```python
from build123d import *

# Parameters (mm, degrees)
F0_W     = 2
F0_H     = 5
F0_W_2   = 47
F0_H_2   = 30
F1_DEPTH = 24
F2_W     = 40
F2_H     = 16
F3_DEPTH = 4
F4_W     = 40
F4_H     = 16
F5_DEPTH = 4
F6_R     = 1.65
F7_DEPTH = 25
F8_R     = 3
F9_DEPTH = 2


with BuildPart() as f1:
    # F0 (on Top) → F1 (new body)
    with BuildSketch(Plane.XY):
        with BuildLine():
            Line((28.5, 14.5), (28.5, 20))
            Line((28.5, 20), (-28.5, 20))
            Line((-28.5, 20), (-28.5, 14.5))
            ThreePointArc((-28.5, 14.5), (-28.646447, 14.146447), (-29, 14))
            Line((-29, 14), (-32.5, 14))
            Line((-32.5, 14), (-32.5, 5))
            Line((-32.5, 5), (-29, 5))
            ThreePointArc((-29, 5), (-28.646447, 4.853553), (-28.5, 4.5))
            Line((-28.5, 4.5), (-28.5, -4.5))
            ThreePointArc((-28.5, -4.5), (-28.646447, -4.853553), (-29, -5))
            Line((-29, -5), (-32.5, -5))
            Line((-32.5, -5), (-32.5, -14))
            Line((-32.5, -14), (-29, -14))
            ThreePointArc((-29, -14), (-28.646447, -14.146447), (-28.5, -14.5))
            Line((-28.5, -14.5), (-28.5, -20))
            Line((-28.5, -20), (28.5, -20))
            Line((28.5, -20), (28.5, -14.5))
            ThreePointArc((28.5, -14.5), (28.646447, -14.146447), (29, -14))
            Line((29, -14), (32.5, -14))
            Line((32.5, -14), (32.5, -5))
            Line((32.5, -5), (29, -5))
            ThreePointArc((29, -5), (28.646447, -4.853553), (28.5, -4.5))
            Line((28.5, -4.5), (28.5, 4.5))
            ThreePointArc((28.5, 4.5), (28.646447, 4.853553), (29, 5))
            Line((29, 5), (32.5, 5))
            Line((32.5, 5), (32.5, 14))
            Line((32.5, 14), (29, 14))
            ThreePointArc((29, 14), (28.646447, 14.146447), (28.5, 14.5))
        make_face()
        with Locations((-29.5, -9.5)):
            Rectangle(F0_W, F0_H, mode=Mode.SUBTRACT)
        with Locations((29.5, -9.5)):
            Rectangle(F0_W, F0_H, mode=Mode.SUBTRACT)
        with Locations((-29.5, 9.5)):
            Rectangle(F0_W, F0_H, mode=Mode.SUBTRACT)
        Rectangle(F0_W_2, F0_H_2, mode=Mode.SUBTRACT)
        with Locations((29.5, 9.5)):
            Rectangle(F0_W, F0_H, mode=Mode.SUBTRACT)
    extrude(amount=F1_DEPTH)

    # F2 (on face) → F3 (cut)
    with BuildSketch(Plane(origin=(-32.5, 0, 0), x_dir=(0, -1, 0), z_dir=(-1, 0, 0))):
        with Locations((0, 12)):
            Rectangle(F2_W, F2_H)
    extrude(amount=-F3_DEPTH, mode=Mode.SUBTRACT)

    # F4 (on face) → F5 (cut)
    with BuildSketch(Plane.YZ.offset(32.5)):
        with Locations((0, 12)):
            Rectangle(F4_W, F4_H)
    extrude(amount=-F5_DEPTH, mode=Mode.SUBTRACT)

    # F6 (on face) → F7 (cut)
    with BuildSketch(Plane.XZ.offset(-15)):
        with Locations((-5, 19)):
            Circle(F6_R)
        with Locations((-5, 5)):
            Circle(F6_R)
        with Locations((5, 19)):
            Circle(F6_R)
        with Locations((5, 5)):
            Circle(F6_R)
    extrude(amount=-F7_DEPTH, mode=Mode.SUBTRACT)

    # F8 (on face) → F9 (cut)
    with BuildSketch(Plane.XZ.offset(-15)):
        with Locations((-5, 19)):
            Circle(F8_R)
        with Locations((-5, 5)):
            Circle(F8_R)
        with Locations((5, 19)):
            Circle(F8_R)
        with Locations((5, 5)):
            Circle(F8_R)
    extrude(amount=-F9_DEPTH, mode=Mode.SUBTRACT)


solid = f1.part
```
Can you work these out from the model? Positions are in its coordinate system, mm. A direction names the side the tool comes from. Round coordinates to 2 decimals unless told otherwise and drop trailing zeros. Loops run counter-clockwise (first coordinate to the right, second up) from the corner with the lowest first, then second, coordinate; pieces in that order, holes last. Notation, with made-up numbers: M 49.5,35.5 L 73.5,35.5 A31 ccw 73.5,72.5 Z; hole C 17.5,-19 d2. An arc over 180 degrees is marked long. Answer as a JSON object with one key per item and string values. Group by question number.
Q1. Imagine slicing it at C-C, the plane y = 11. Please give me the cut outline in (x, z), then the cut area to 3 significant figures.
Q2. On a 3-axis mill with a long thin cutter (end or side, diameter ignored), from which of +Z, -Z, +X, -X, +Y, -Y can I reach the whole of each face in a straight line? I mean faces 1 (the flat face through (30.5, 9, 22)), 2 (the flat face through (-31, 5, 2)), 3 (the cylindrical face through (-3.616, 15.986, 2.338)), 4 (the flat face through (31, -5, 22)). Say none if no direction works.
Q3. Imagine slicing it at D-D, the plane z = 9. Please give me the cut outline in (x, y).
Q4. Please list where these lines run through material, in increasing order: L1, parallel to X at y = -8, z = 3.25; L2, parallel to Z at x = 5, y = 15.8; L3, parallel to X at y = -14, z = 10.75.
Q5. Imagine slicing it at A-A, the plane z = 5. Please give me the cut outline in (x, y).
Q6. Imagine slicing it at B-B, the plane x = -16.5. Please give me the cut outline in (y, z), then the cut area to 3 significant figures.
Q7. Will these pins go through, and if not, where does the flat tip stop? pin 1 (1 mm diameter, centred on x = -30, z = 2, fed in from -Y); pin 2 (6 mm diameter, centred on y = 15, z = 10.5, fed in from -X); pin 3 (6 mm diameter, centred on y = -2, z = 10, fed in from +X).
Q8. We'd pull the mould along Z, two halves only. Please class faces 5 (the flat face through (31, 14, 22)), 6 (the flat face through (31, 11, 20)): +Z half, -Z half, draft (parallel to the pull), parting line (faces both ways), or undercut.
Findings:
{
 "1": {"outline": "M -32.5,0 L -30.5,0 L -30.5,4 L -32.5,4 Z; M -32.5,20 L -30.5,20 L -30.5,24 L -32.5,24 Z; M -28.5,0 L -23.5,0 L -23.5,24 L -28.5,24 Z; M 23.5,0 L 28.5,0 L 28.5,24 L 23.5,24 Z; M 30.5,0 L 32.5,0 L 32.5,4 L 30.5,4 Z; M 30.5,20 L 32.5,20 L 32.5,24 L 30.5,24 Z", "area": "272 mm2"},
 "2": {"face 1": "+Z, -Z", "face 2": "+Z, -Z, -X", "face 3": "none", "face 4": "+Z, -Z, +X"},
 "3": {"outline": "M -28.5,-20 L 28.5,-20 L 28.5,20 L -28.5,20 Z; hole M -23.5,-15 L 23.5,-15 L 23.5,15 L -23.5,15 Z"},
 "4": {"L1": "x = -32.5 to -30.5, -28.5 to -23.5, 23.5 to 28.5, 30.5 to 32.5", "L2": "z = 0 to 2, 8 to 16, 22 to 24", "L3": "x = -28.5 to -23.5, 23.5 to 28.5"},
 "5": {"outline": "M -28.5,-20 L 28.5,-20 L 28.5,20 L 6.65,20 L 6.65,17 L 8,17 L 8,15 L 23.5,15 L 23.5,-15 L -23.5,-15 L -23.5,15 L -8,15 L -8,17 L -6.65,17 L -6.65,20 L -28.5,20 Z; M -3.35,17 L -2,17 L -2,15 L 2,15 L 2,17 L 3.35,17 L 3.35,20 L -3.35,20 Z"},
 "6": {"outline": "M -20,0 L -15,0 L -15,24 L -20,24 Z; M 15,0 L 20,0 L 20,24 L 15,24 Z", "area": "240 mm2"},
 "7": {"pin 1": "stops at y = -14", "pin 2": "stops at x = -28.5", "pin 3": "stops at x = 28.5"},
 "8": {"face 5": "draft", "face 6": "undercut"}
}
